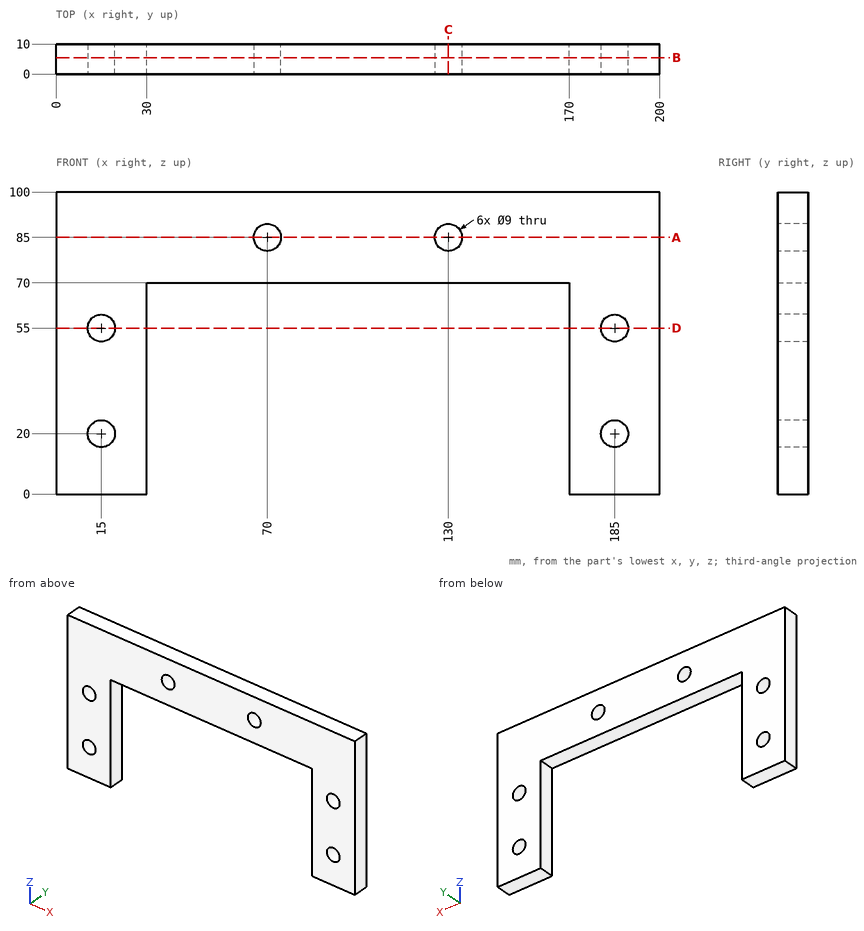
Study the drawing (mm; zero at the part's minimum x, y, z) and answer. Coordinates: 2 decimals unless noted, no trailing zeros. Write each loop counter-clockwise with the first axis right and the second up, starting at its lowest first coordinate (ties: lowest second). Pieces come first, ordered by that corner, then holes. Notation, with made-up numbers: (52, 78.25) - (98, 78.25) arc R23 ccw to (98, 101.25) - close; hole circle Ø9 at (-31.75, 7). An arc over 180 degrees is marked (long way). One line per item, written item: value.
1) Find section B-B (y = 5.5). Give the vertices of the cut face in (x, z), and give its area (3 significant figures).
Geometry check:
outline: (0, 0) - (30, 0) - (30, 70) - (170, 70) - (170, 0) - (200, 0) - (200, 100) - (0, 100) - close; hole circle Ø9 at (15, 20); hole circle Ø9 at (15, 55); hole circle Ø9 at (70, 85); hole circle Ø9 at (130, 85); hole circle Ø9 at (185, 20); hole circle Ø9 at (185, 55)
area: 9,820 mm2
2) Consider line 1 along X through (y, z) = (2.5, 55); line 2 along Z through (x, y) = (15, 7); line 3 along Z through (x, y) = (130, 4). Determine where each line is inside the solid, lowest interval first. Write a range as from..to.
Geometry check:
line 1: x = 0..10.5, 19.5..30, 170..180.5, 189.5..200
line 2: z = 0..15.5, 24.5..50.5, 59.5..100
line 3: z = 70..80.5, 89.5..100
3) Find section A-A (z = 85). Give the vertices of the cut face in (x, y).
Geometry check:
outline: (0, 0) - (65.5, 0) - (65.5, 10) - (0, 10) - close; (74.5, 0) - (125.5, 0) - (125.5, 10) - (74.5, 10) - close; (134.5, 0) - (200, 0) - (200, 10) - (134.5, 10) - close
4) Find section C-C (x = 130). Give the vertices of the cut face in (y, z), and give its area (3 significant figures).
Geometry check:
outline: (0, 70) - (10, 70) - (10, 80.5) - (0, 80.5) - close; (0, 89.5) - (10, 89.5) - (10, 100) - (0, 100) - close
area: 210 mm2
5) Each of these flat-tipped pins is pushed along its axis until it touches: pin 1 Ø7 at (x, z) = (130, 85) entering from -Y; pin 2 Ø5 at (x, y) = (114.5, 4.5) entering from -Z. Where does it stop, or does it pass through?
Geometry check:
pin 1: passes through
pin 2: stops at z = 70
6) Find section D-D (z = 55). Give the vertices of the cut face in (x, y), and give its area (3 significant figures).
Geometry check:
outline: (0, 0) - (10.5, 0) - (10.5, 10) - (0, 10) - close; (19.5, 0) - (30, 0) - (30, 10) - (19.5, 10) - close; (170, 0) - (180.5, 0) - (180.5, 10) - (170, 10) - close; (189.5, 0) - (200, 0) - (200, 10) - (189.5, 10) - close
area: 420 mm2
